Model file for the job. Use its own axes, mm. A direction names the side the tool comes from. Give positions to 0.01 mm unless a question says otherwise; leave off trailing zeros. Order: outer loops, then holes, each group sorted by start corner. A loop starts at its lowest first (then second) coordinate and runs counter-clockwise, first axis right, second up. Notation, with made-up numbers: M 74,13.5 L 115,13.5 A17 ccw 115,39.5 Z; hole C -11.75,60.25 d10. An arc over 180 degrees is marked long. Return JSON: item names as keys, results as strings. Group by question number.
1. Slice it at A-A on z = 3.75. Give the number of separate pieces and of enclosed holes in the cut face, then the cut area to 3 significant figures.
2. Slice it at C-C on z = 14.75. List the corners of the cut face in (x, y) (3 decimals).
3. Wall check: probe 1 along Y at (x, z) = (0, 2.1); probe 2 along Y at (x, z) = (0, 1.6); probe 3 along Z at (x, y) = (18, -13.5). Give the ranges that are in metal, low to high. Write a range as [from, to].
4. Pin check, flat tips, straight feed: pin 1 (12.5 mm diameter, centred on x = 6, y = 1.5, fed in from +Z); pin 2 (1.5 mm diameter, centred on x = 11, z = 16, fed in from +Y); pin 3 (1 mm diameter, centred on y = 20.5, z = 9.5, fed in from -X). Stop position of each tip, or through.
5. 3-axis set-ups, long thin cutter, end or side, ignore diameter. For faces 1 (the face through (0, 27, 16.51)), 2 (the face through (-0.33, 2.52, 1.16)), 3 (the face through (-3.48, -1.97, 3.96)): which of +Z, -Z, +X, -X, +Y, -Y reach the whole face in a straight line?
6. Two-plate mould, pull along Y, no slides. Class faces 4 (the face through (0, 27, 12.7)), 5 (the face through (13.77, -26.48, 11.97)), 6 (the face through (-3.448, 2.028, 3.96)), 7 (the face through (3.48, 1.97, 3.96)): released by +Y, released by -Y, zero draft, split by the parting line, or undercut.
from build123d import *

# Parameters (mm, degrees)
F0_R      = 29.845
F1_DEPTH  = 21.59
F2_R      = 26.797
F3_DEPTH  = 10.16
F3_TAPER  = 2
F4_R      = 23.8125
F5_DEPTH  = 8.89
F6_R      = 6.35
F7_DEPTH  = 3.048
F8_R      = 2.54
F9_DEPTH  = 25.4
F12_DEPTH = 3.302
F13_R     = 5.08
F14_R     = 2.54
F15_R     = 19.05
F15_R_2   = 12.7
F16_DEPTH = 1.27
F18_DEPTH = 8.89
F19_R     = 1.4605
F20_DEPTH = 1.905
F21_R     = 1.27
F22_W     = 7.62
F22_H     = 3.81
F23_DEPTH = 36.576
F25_DEPTH = 16.51
F27_DEPTH = 19.0510001
F29_W     = 11.43
F29_H     = 7.62
F30_DEPTH = 3.81


with BuildPart() as f1:
    # F0 (on Top) → F1 (new body)
    with BuildSketch(Plane.XY):
        Circle(F0_R)
    extrude(amount=F1_DEPTH)

    # F2 (on face) → F3 (cut)
    with BuildSketch(Plane.XY.offset(21.59)):
        Circle(F2_R)
    extrude(amount=-F3_DEPTH, taper=F3_TAPER, mode=Mode.SUBTRACT)

    # F4 (on face) → F5 (cut)
    with BuildSketch(Plane.XY.offset(11.43)):
        Circle(F4_R)
    extrude(amount=-F5_DEPTH, mode=Mode.SUBTRACT)

    # F6 (on face) → F7 (join)
    with BuildSketch(Plane.XY.offset(2.54)):
        Circle(F6_R)
    extrude(amount=F7_DEPTH)

    # F8 (on face) → F9 (cut)
    with BuildSketch(Plane.XY.offset(5.588)):
        Circle(F8_R)
    extrude(amount=-F9_DEPTH, mode=Mode.SUBTRACT)

    # F11 (on offset) → F12 (cut)
    with BuildSketch(Plane.XY.offset(5.588)):
        Polygon((-2.3096897519, -4.0005), (2.3096897519, -4.0005), (4.6193795038, 0), (2.3096897519, 4.0005), (-2.3096897519, 4.0005), (-4.6193795038, 0), align=None)
    extrude(amount=-F12_DEPTH, mode=Mode.SUBTRACT)

    # F13
    f13_edges = [f1.edges().sort_by_distance(p)[0] for p in [
        (-29.845, 0, 0),
    ]]
    fillet(f13_edges, radius=F13_R)

    # F14
    f14_edges = [f1.edges().sort_by_distance(p)[0] for p in [
        (-29.845, 0, 21.59),
    ]]
    fillet(f14_edges, radius=F14_R)

    # F15 (on face) → F16 (cut)
    with BuildSketch(Plane.XY.offset(2.54)):
        Circle(F15_R)
        Circle(F15_R_2, mode=Mode.SUBTRACT)
    extrude(amount=-F16_DEPTH, mode=Mode.SUBTRACT)

    # F17 (on face) → F18 (join, through all)
    with BuildSketch(Plane.XY.offset(2.54)):
        with BuildLine():
            Line((-19.05, 0), (-19.05, 14.2875))
            ThreePointArc((-19.05, 14.2875), (-23.8125, 0), (-19.05, -14.2875))
            Line((-19.05, -14.2875), (-19.05, 0))
        make_face()
        with BuildLine():
            ThreePointArc((23.8125, 0), (22.5905210348, 7.5301736783), (19.05, 14.2875))
            Line((19.05, 14.2875), (19.05, 0))
            Line((19.05, 0), (19.05, -14.2875))
            ThreePointArc((19.05, -14.2875), (22.5905210348, -7.5301736783), (23.8125, 0))
        make_face()
    extrude(amount=F18_DEPTH)

    # F19 (on face) → F20 (join)
    with BuildSketch(Plane.XY.offset(11.43)):
        with Locations((-22.86, 0.508)):
            Circle(F19_R)
        with Locations((22.86, 0.508)):
            Circle(F19_R)
    extrude(amount=F20_DEPTH)

    # F21
    f21_edges = [f1.edges().sort_by_distance(p)[0] for p in [
        (-24.3205, 0.508, 13.335),
        (21.3995, 0.508, 13.335),
    ]]
    fillet(f21_edges, radius=F21_R)

    # F22 (on Front) → F23 (cut)
    with BuildSketch(Plane.XZ):
        with Locations((0, 14.605)):
            Rectangle(F22_W, F22_H)
    extrude(amount=-F23_DEPTH, mode=Mode.SUBTRACT)

    # F24 (on face) → F25 (cut)
    with BuildSketch(Plane.XY.offset(21.59)):
        with BuildLine():
            ThreePointArc((-3.39725, -26.5807806777), (0, -26.797), (3.39725, -26.5807806777))
            Line((3.39725, -26.5807806777), (3.39725, -23.129734925))
            Line((3.39725, -23.129734925), (-3.39725, -23.129734925))
            Line((-3.39725, -23.129734925), (-3.39725, -26.5807806777))
        make_face()
        with BuildLine():
            Line((-3.39725, -28.209734925), (3.39725, -28.209734925))
            Line((3.39725, -28.209734925), (3.39725, -27.0928351679))
            ThreePointArc((3.39725, -27.0928351679), (0, -27.305), (-3.39725, -27.0928351679))
            Line((-3.39725, -27.0928351679), (-3.39725, -28.209734925))
        make_face()
        with BuildLine():
            ThreePointArc((-3.39725, -27.0928351679), (0, -27.305), (3.39725, -27.0928351679))
            Line((3.39725, -27.0928351679), (3.39725, -26.5807806777))
            ThreePointArc((3.39725, -26.5807806777), (0, -26.797), (-3.39725, -26.5807806777))
            Line((-3.39725, -26.5807806777), (-3.39725, -27.0928351679))
        make_face()
    extrude(amount=-F25_DEPTH, mode=Mode.SUBTRACT)

    # F26 (on face) → F27 (cut, through all)
    with BuildSketch(Plane.XY.offset(2.54)):
        with BuildLine():
            ThreePointArc((19.05, -14.2875), (0, -23.8125), (-19.05, -14.2875))
            Line((-19.05, -14.2875), (-19.05, -16.3165347501))
            ThreePointArc((-19.05, -16.3165347501), (0, -25.0825), (19.05, -16.3165347501))
            Line((19.05, -16.3165347501), (19.05, -14.2875))
        make_face()
    extrude(amount=F27_DEPTH, mode=Mode.SUBTRACT)

    # F29 (on offset) → F30 (cut)
    with BuildSketch(Plane.XZ.offset(-31.75)):
        with Locations((0, 14.605)):
            Rectangle(F29_W, F29_H)
    extrude(amount=F30_DEPTH, mode=Mode.SUBTRACT)


solid = f1.part
Result:
{
 "1": {"separate pieces": "2", "enclosed holes": "2", "area": "1,180 mm2"},
 "2": {"outline": "M -5.715,27.94 L -5.715,29.293 A29.845 ccw long 5.715,29.293 L 5.715,27.94 L 3.81,27.94 L 3.81,26.283 A26.558 cw 3.397,-26.34 L 3.397,-28.21 L -3.397,-28.21 L -3.397,-26.34 A26.558 cw -3.81,26.283 L -3.81,27.94 Z"},
 "3": {"probe 1": "y = [-28.88, -19.05], [-12.7, -2.54], [2.54, 12.7], [19.05, 28.88]", "probe 2": "y = [-28.47, -19.05], [-12.7, -2.54], [2.54, 12.7], [19.05, 28.47]", "probe 3": "z = [0, 2.54]"},
 "4": {"pin 1": "stops at z = 5.59", "pin 2": "stops at y = 28.03", "pin 3": "stops at x = -22.15"},
 "5": {"face 1": "+Y", "face 2": "+Z, -Z", "face 3": "+Z"},
 "6": {"face 4": "zero draft", "face 5": "split by the parting line", "face 6": "undercut", "face 7": "undercut"}
}
